Design review of the part shown in the three views and the two pictorial views. Dimensions are in mm from the part's minimum x, y and z. A direction names the side the tool comes from. Round coordinates to 2 decimals unless told otherwise and drop trailing zeros. Loops run counter-clockwise (first coordinate to the right, second up) from the corner with the lowest first, then second, coordinate; pieces in that order, holes last. Notation, with made-up numbers: M 15,42 L 33,42 A22 ccw 33,61 Z; hole C 76,-25 d9. An arc over 180 degrees is marked long. One line per question, with ' | ' between items.
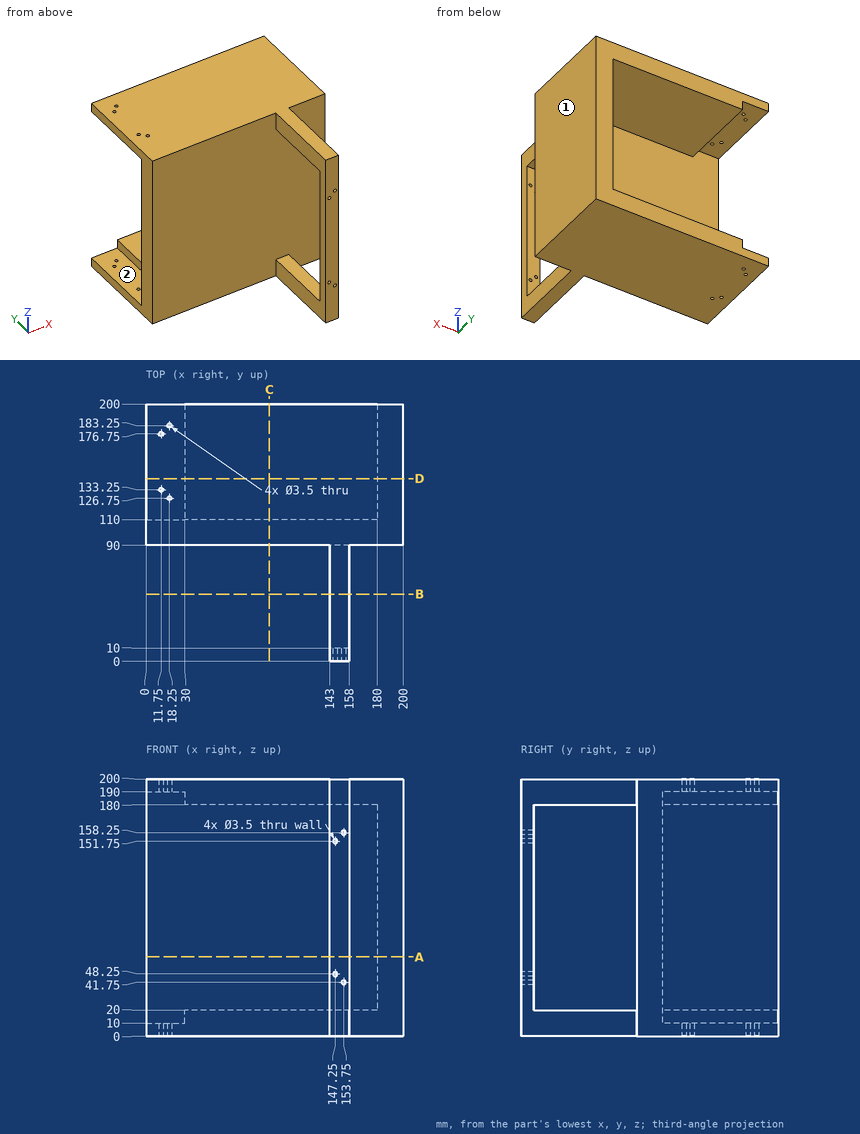
1) Add section C-C on x = 96. State the section outline as (y, z) points, then the cut area to 3 significant figures.
Output values:
outline: M 90,0 L 200,0 L 200,20 L 110,20 L 110,180 L 200,180 L 200,200 L 90,200 Z | area: 7,600 mm²
2) Insertion check: P1, Ø10, axis at y = 82.5, z = 131.5, coming from the -X side (3 decimals); P2, Ø5.5, axis at x = 153.75, z = 158.25, coming from the +Y side; P3, Ø5, axis at x = 74, z = 145, coming from the -Y side; P4, Ø12, axis at y = 136, z = 126.5, coming from the -X side. Each pin has a flat end and moves straight along its axis. Give the tip position at first contact, or say it passes through.
Output values:
P1: passes through | P2: stops at y = 110 | P3: stops at y = 90 | P4: stops at x = 180
3) Add section D-D on y = 142. State the section outline as (x, z) points, then the cut area to 3 significant figures.
Output values:
outline: M 0,0 L 200,0 L 200,200 L 0,200 L 0,190 L 30,190 L 30,180 L 180,180 L 180,20 L 30,20 L 30,10 L 0,10 Z | area: 10,600 mm²
4) Machinability: for the marked faces 1 and 2, which of the approach directions +Z, -Z, +X, -X, +Y, -Y give a long, thin tool a straight path to every point of the face, cutting with its end or side? Answer none if there is none.
Output values:
face 1: +Z, -Z, +X, +Y, -Y | face 2: -X, +Y
5) For line 1 (Y direction, x = 11.75, z = 193.75); line 2 (X direction, y = 176.75, z = 192); line 3 (Z direction, x = 147, y = 5), list the stretches that pass through material, from the lowest coordinate up.
Output values:
line 1: y = 90 to 131.5, 135 to 175, 178.5 to 200 | line 2: x = 0 to 10, 13.5 to 200 | line 3: z = 0 to 46.52, 49.98 to 150.02, 153.48 to 200
6) Add section A-A on z = 61.5. State the section outline as (x, y) points, then the cut area to 3 significant figures.
Output values:
outline: M 0,90 L 200,90 L 200,200 L 180,200 L 180,110 L 0,110 Z; M 143,0 L 158,0 L 158,10 L 143,10 Z | area: 5,950 mm²
7) Add section B-B on y = 52. State the section outline as (x, z) points, then the cut area to 3 significant figures.
Output values:
outline: M 143,0 L 158,0 L 158,20 L 143,20 Z; M 143,180 L 158,180 L 158,200 L 143,200 Z | area: 600 mm²
